Verification items for the finished model (mm, model axes). Face numbers are marked on the shaded views. Give positions to 0.01 mm unless a question says otherwise; leave off trailing zeros. Order: outer loops, then holes, each group sorted by start corner. A loop starts at its lowest first (then second) coordinate and runs counter-clockwise, first axis right, second up. Notation, with made-up numbers: M 32.5,74.25 L 38.5,74.25 A16 cw 38.5,101.25 Z; hole C 66.5,56.25 d2. An arc over 180 degrees is marked long. Answer as a JSON object with one key per item and string values.
```python
from build123d import *

# Parameters (mm, degrees)
ESQUISSE5_R                  = 24
ESQUISSE5_R_2                = 14.5
BOSS_EXTRU_2_DEPTH           = 50
ENL_V_MAT_EXTRU_4_DEPTH      = 51
ENL_V_MAT_EXTRU_4_DEPTH_BACK = 16


with BuildPart() as part:
    # Esquisse5 → Boss.-Extru.2 (new body)
    with BuildSketch(Plane.XY):
        Circle(ESQUISSE5_R)
        Circle(ESQUISSE5_R_2, mode=Mode.SUBTRACT)
    extrude(amount=BOSS_EXTRU_2_DEPTH)

    # Esquisse6 → Enlèv. mat.-Extru.4 (cut, two sides)
    with BuildSketch(Plane.XY) as enl_v_mat_extru_4_sk:
        with BuildLine():
            Line((-4.384096163, 23.596179793), (-5.367769198, 20.017709679))
            ThreePointArc((-5.367769198, 20.017709679), (0, 20.724904028), (5.367769198, 20.017709679))
            Line((5.367769198, 20.017709679), (4.384096163, 23.596179793))
            ThreePointArc((4.384096163, 23.596179793), (0, 24), (-4.384096163, 23.596179793))
        make_face()
        with BuildLine():
            Line((19.785042868, 13.584994616), (17.950244258, 10.359072259))
            ThreePointArc((17.950244258, 10.359072259), (14.654720178, 14.654720178), (10.359072259, 17.950244258))
            Line((10.359072259, 17.950244258), (13.584994616, 19.785042868))
            ThreePointArc((13.584994616, 19.785042868), (16.970562748, 16.970562748), (19.785042868, 13.584994616))
        make_face()
        with BuildLine():
            Line((23.596179793, -4.384096163), (20.017709679, -5.367769198))
            ThreePointArc((20.017709679, -5.367769198), (20.724904028, 0), (20.017709679, 5.367769198))
            Line((20.017709679, 5.367769198), (23.596179793, 4.384096163))
            ThreePointArc((23.596179793, 4.384096163), (24, 0), (23.596179793, -4.384096163))
        make_face()
        with BuildLine():
            Line((13.584994616, -19.785042868), (10.359072259, -17.950244258))
            ThreePointArc((10.359072259, -17.950244258), (14.654720178, -14.654720178), (17.950244258, -10.359072259))
            Line((17.950244258, -10.359072259), (19.785042868, -13.584994616))
            ThreePointArc((19.785042868, -13.584994616), (16.970562748, -16.970562748), (13.584994616, -19.785042868))
        make_face()
        with BuildLine():
            Line((-4.384096163, -23.596179793), (-5.367769198, -20.017709679))
            ThreePointArc((-5.367769198, -20.017709679), (0, -20.724904028), (5.367769198, -20.017709679))
            Line((5.367769198, -20.017709679), (4.384096163, -23.596179793))
            ThreePointArc((4.384096163, -23.596179793), (0, -24), (-4.384096163, -23.596179793))
        make_face()
        with BuildLine():
            Line((-19.785042868, -13.584994616), (-17.950244258, -10.359072259))
            ThreePointArc((-17.950244258, -10.359072259), (-14.654720178, -14.654720178), (-10.359072259, -17.950244258))
            Line((-10.359072259, -17.950244258), (-13.584994616, -19.785042868))
            ThreePointArc((-13.584994616, -19.785042868), (-16.970562748, -16.970562748), (-19.785042868, -13.584994616))
        make_face()
        with BuildLine():
            Line((-23.596179793, 4.384096163), (-20.017709679, 5.367769198))
            ThreePointArc((-20.017709679, 5.367769198), (-20.724904028, 0), (-20.017709679, -5.367769198))
            Line((-20.017709679, -5.367769198), (-23.596179793, -4.384096163))
            ThreePointArc((-23.596179793, -4.384096163), (-24, 0), (-23.596179793, 4.384096163))
        make_face()
        with BuildLine():
            Line((-13.584994616, 19.785042868), (-10.359072259, 17.950244258))
            ThreePointArc((-10.359072259, 17.950244258), (-14.654720178, 14.654720178), (-17.950244258, 10.359072259))
            Line((-17.950244258, 10.359072259), (-19.785042868, 13.584994616))
            ThreePointArc((-19.785042868, 13.584994616), (-16.970562748, 16.970562748), (-13.584994616, 19.785042868))
        make_face()
    extrude(amount=ENL_V_MAT_EXTRU_4_DEPTH, mode=Mode.SUBTRACT)
    extrude(enl_v_mat_extru_4_sk.sketch, amount=-ENL_V_MAT_EXTRU_4_DEPTH_BACK, mode=Mode.SUBTRACT)


solid = part.part
```
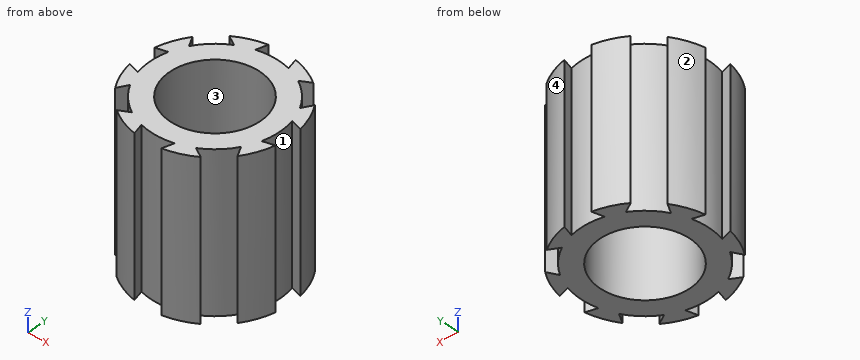
Q1. Section check A-A on x = 0. Record the cut outline in (y, z), then the cut area to 3 significant figures.
Resolved:
{"outline": "M -20.72,0 L -14.5,0 L -14.5,50 L -20.72,50 Z; M 14.5,0 L 20.72,0 L 20.72,50 L 14.5,50 Z", "area": "622 mm²"}
Q2. Material ranges on L1, parallel to Y at x = 13, z = 44; L2, parallel to Y at x = 0, z = 39; L3, parallel to Y at x = -12.5, z = 35.5, recorded low to high.
Resolved:
{"L1": "y = -20.17 to -19.45, -16.14 to -6.42, 6.42 to 16.14, 19.45 to 20.17", "L2": "y = -20.72 to -14.5, 14.5 to 20.72", "L3": "y = -20.49 to -19.17, -16.53 to -7.35, 7.35 to 16.53, 19.17 to 20.49"}
Q3. Gauge pin test, flat ends, axial feed: pin 1 Ø8 at (x, z) = (-14, 18) entering from +Y; pin 2 Ø1 at (x, z) = (-18.5, 21.5) entering from -Y; pin 3 Ø2 at (y, z) = (3, 11) entering from +X. Record the tip position at first contact, or that the pin passes through.
Resolved:
{"pin 1": "stops at y = 21.82", "pin 2": "stops at y = -12.2", "pin 3": "stops at x = 20.63"}
Q4. Section check D-D on x = 15.5. Record the cut outline in (y, z).
Resolved:
{"outline": "M -13.76,0 L 13.76,0 L 13.76,50 L -13.76,50 Z"}
Q5. Release check for a two-part mould opening along X. For the marked faces 1, 2, 3 and 4 record: +X half, -X half, draft (parallel to the pull), parting line (faces both ways), or undercut.
Resolved:
{"face 1": "undercut", "face 2": "-X half", "face 3": "undercut", "face 4": "+X half"}
